Autodesk Inventor part; units mm, degrees
ref_plane "p1_XY" through (0, 0, 2.3749) normal (1, 0, 0) x (0, 0, -1)
ref_plane "p1_YZ" through (0, 0, 2.3749) normal (0, 0, -1) x (0, 1, 0)
ref_plane "p1_ZX" through (0, 0, 2.3749) normal (0, 1, 0) x (1, 0, 0)
sketch "Sketch_1" plane through (0, 0, 0) normal (0, 0, 1) x (1, 0, 0)
  line L0 (6.9342, 0) -> (-6.9342, 0)
  line L1 (-6.9342, 0) -> (-6.9342, 1.9939)
  line L2 (-6.9342, 1.9939) -> (-6.5532, 2.3749)
  line L3 (-6.5532, 2.3749) -> (-5.6007, 2.3749)
  line L4 (-5.6007, 2.3749) -> (-5.6007, 1.8796)
  line L5 (-5.6007, 1.8796) -> (-4.826, 1.8796)
  line L6 (-4.826, 1.8796) -> (-4.826, 2.3749)
  line L7 (-4.826, 2.3749) -> (4.826, 2.3749)
  line L8 (4.826, 2.3749) -> (4.826, 1.8796)
  line L9 (4.826, 1.8796) -> (5.6007, 1.8796)
  line L10 (5.6007, 1.8796) -> (5.6007, 2.3749)
  line L11 (5.6007, 2.3749) -> (6.5532, 2.3749)
  line L12 (6.5532, 2.3749) -> (6.9342, 1.9939)
  line L13 (6.9342, 1.9939) -> (6.9342, 0)
  line L14 (6.9342, 0) -> (-6.9342, 0)
revolve "Revolution1" add sketch "Sketch_1" angle 360 about axis through (6.9342, 0, 0) along (1, 0, 0)
ref_plane "p1_XY" through (0, 0, 2.3749) normal (1, 0, 0) x (0, 0, -1)
ref_plane "p1_YZ" through (0, 0, 2.3749) normal (0, 0, -1) x (0, 1, 0)
ref_plane "p1_ZX" through (0, 0, 2.3749) normal (0, 1, 0) x (1, 0, 0)
ref_plane "p2_XY" through (0, 0, -2.3749) normal (1, 0, 0) x (0, 0, -1)
ref_plane "p2_YZ" through (0, 0, -2.3749) normal (0, 0, -1) x (0, 1, 0)
ref_plane "p2_ZX" through (0, 0, -2.3749) normal (0, 1, 0) x (1, 0, 0)
ref_plane "pin_XY" through (0, 0, 0) normal (1, 0, 0) x (0, 0, -1)
ref_plane "pin_YZ" through (0, 0, 0) normal (0, 0, -1) x (0, 1, 0)
ref_plane "pin_ZX" through (0, 0, 0) normal (0, 1, 0) x (1, 0, 0)
ref_plane "rr1_XY" through (5.2134, 0, 0) normal (1, 0, 0) x (0, 0, -1)
ref_plane "rr1_YZ" through (5.2134, 0, 0) normal (0, 0, -1) x (0, 1, 0)
ref_plane "rr1_ZX" through (5.2134, 0, 0) normal (0, 1, 0) x (1, 0, 0)
ref_plane "rr2_XY" through (-5.2134, 0, 0) normal (1, 0, 0) x (0, 0, -1)
ref_plane "rr2_YZ" through (-5.2134, 0, 0) normal (0, 0, -1) x (0, 1, 0)
ref_plane "rr2_ZX" through (-5.2134, 0, 0) normal (0, 1, 0) x (1, 0, 0)
ref_plane "w21_XY" through (6.9342, 0, 0) normal (0, 1, 0) x (1, 0, 0)
ref_plane "w21_YZ" through (6.9342, 0, 0) normal (1, 0, 0) x (0, 0, -1)
ref_plane "w21_ZX" through (6.9342, 0, 0) normal (0, 0, -1) x (0, 1, 0)
ref_plane "w22_XY" through (-6.9342, 0, 0) normal (0, 1, 0) x (1, 0, 0)
ref_plane "w22_YZ" through (-6.9342, 0, 0) normal (1, 0, 0) x (0, 0, -1)
ref_plane "w22_ZX" through (-6.9342, 0, 0) normal (0, 0, -1) x (0, 1, 0)
properties part number "D-12304"
Geometry check sheet. Reference: the model listing, model coordinates, mm. Give positions to 0.01 mm unless a question says otherwise; leave off trailing zeros. Loops run counter-clockwise (first coordinate to the right, second up) from the corner with the lowest first, then second, coordinate; pieces in that order, holes last. Notation, with made-up numbers: (82.25, 72.25) - (131.25, 72.25) arc R26 ccw to (131.25, 110.25) - close; hole circle Ø5 at (-19.75, -30). An arc over 180 degrees is marked (long way). Use CSV: the item, a comma, the result in double quotes. Start each with the question number.
Q1. Section check A-A, the plane y = 0. Record the cut outline in (x, z), and give its area (3 significant figures).
Q2. Section check B-B, the plane x = 1.5. Record the cut outline in (y, z).
Q3. Release check for a two-part mould opening along X. For faces 1 (the face through (5.219, -0.407, -1.835)), 2 (the face through (-5.208, -0.407, -1.835)), 3 (the face through (6.934, 0, 0)), 4 (the face through (-6.07, -1.75, 1.605)) record: +X half, -X half, draft (parallel to the pull), parting line (faces both ways), or undercut.
Q4. Scan lines: probe 1 along X at (y, z) = (-1.95, -1.15); probe 2 along Y at (x, z) = (-0.5, -1.45); probe 3 along Z at (x, y) = (6.25, 1.9). Record each from-to range of solid material in increasing order. Write a range as from..to.
Findings below:
1,outline,"(-6.93, -1.99) - (-6.55, -2.37) - (-5.6, -2.37) - (-5.6, -1.88) - (-4.83, -1.88) - (-4.83, -2.37) - (4.83, -2.37) - (4.83, -1.88) - (5.6, -1.88) - (5.6, -2.37) - (6.55, -2.37) - (6.93, -1.99) - (6.93, 1.99) - (6.55, 2.37) - (5.6, 2.37) - (5.6, 1.88) - (4.83, 1.88) - (4.83, 2.37) - (-4.83, 2.37) - (-4.83, 1.88) - (-5.6, 1.88) - (-5.6, 2.37) - (-6.55, 2.37) - (-6.93, 1.99) - close"
1,area,"64.0 mm^2"
2,outline,"circle Ø4.75 at (0, 0)"
3,face 1,"undercut"
3,face 2,"undercut"
3,face 3,"+X half"
3,face 4,"draft"
4,probe 1,"x = -6.66..-5.6, -4.83..4.83, 5.6..6.66"
4,probe 2,"y = -1.88..1.88"
4,probe 3,"z = -1.42..1.42"
